from build123d import *

# Parameters (mm, degrees)
SKETCH_1_R      = 17.5
EXTRUDE_1_DEPTH = 10
SKETCH_2_R      = 15
EXTRUDE_2_DEPTH = 300
SKETCH_3_R      = 75
EXTRUDE_3_DEPTH = 10
FILLET_1_R      = 10
HOLE_WIZARD_1_D = 24


with BuildPart() as part:
    # 草图1 → 凸台-拉伸1 (new body)
    with BuildSketch(Plane(origin=(0, 0, 0), x_dir=(1, 0, 0), z_dir=(0, 1, 0))):
        with Locations(Location((0, 0, 0), (0, 0, 270))):
            Circle(SKETCH_1_R)
    extrude(amount=EXTRUDE_1_DEPTH)

    # 草图2 → 凸台-拉伸2 (add)
    with BuildSketch(Plane(origin=(0, 0, 0), x_dir=(1, 0, 0), z_dir=(0, 1, 0))):
        with Locations(Location((0, 0, 0), (0, 0, 270))):
            Circle(SKETCH_2_R)
    extrude(amount=EXTRUDE_2_DEPTH)

    # 草图3 → 凸台-拉伸3 (add)
    with BuildSketch(Plane(origin=(0, 300, 0), x_dir=(1, 0, 0), z_dir=(0, 1, 0))):
        with Locations(Location((0, 0, 0), (0, 0, 270))):
            Circle(SKETCH_3_R)
    extrude(amount=EXTRUDE_3_DEPTH)

    # 圆角1
    fillet_1_edges = [part.edges().sort_by_distance(p)[0] for p in [
        (0, 300, -15),
    ]]
    fillet(fillet_1_edges, radius=FILLET_1_R)

    # 孔1 (through all)
    with Locations(Plane(origin=(0, 310, 0), x_dir=(1, 0, 0), z_dir=(0, 1, 0))):
        with Locations((0, 50), (50, 0), (0, -50), (-50, 0)):
            Hole(HOLE_WIZARD_1_D / 2)


solid = part.part
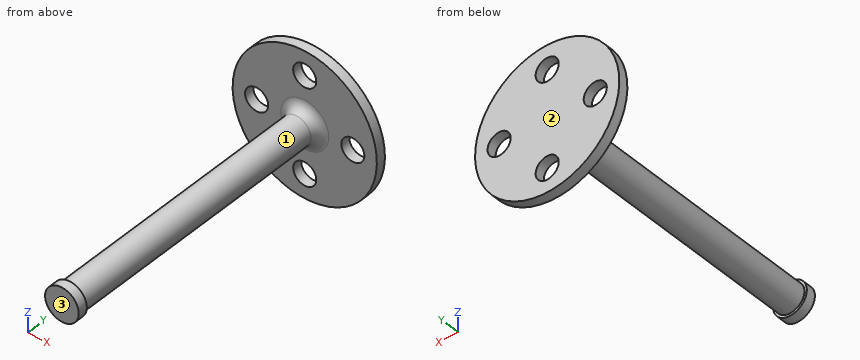
Geometry: final body of the model. Coordinates: model frame, mm. Face numbers are marked on the shaded views. Round coordinates to 2 decimals unless told otherwise and drop trailing zeros. Loops run counter-clockwise (first coordinate to the right, second up) from the corner with the lowest first, then second, coordinate; pieces in that order, holes last. Notation, with made-up numbers: (3.5, -25) - (20.5, -25) arc R12 ccw to (20.5, -14) - close; hole circle Ø7 at (-21.75, -13). An arc over 180 degrees is marked (long way). Write each question's results on one line, items separated by ' | '. Start each with the question number.
1) Mould query, pull axis Y, two halves, no side actions, for the marked faces 1, 2 and 3. Classes: released by +Y, released by -Y, zero draft, split by the parting line, or undercut.
2) Line query: probe 1 along Y at (x, z) = (-25.5, 27.5); probe 2 along X at (y, z) = (164, 1); probe 3 along Z at (x, y) = (-50, 305.5). Output: solid intervals per line, ascending. Write a range as [from, to].
3) Cut plane C-C on x = -50. Return loops of the section in (y, z), then the cut area to 3 significant figures.
4) Cut plane A-A on z = 0. Return loops of the section in (x, y), then the cut area to 3 significant figures.
5) First-contact query: P1, Ø1.5, axis at y = 92, z = -7, coming from the -X side; P2, Ø1.5, axis at x = -4.5, z = 9.5, coming from the -Y side. Flat tips, straight axial feed; report the tip coordinate or a pass-through.
6) Cut plane D-D on z = 50. Return loops of the section in (x, y), then the cut area to 3 significant figures.
7) Cut plane B-B on x = 0. Return loops of the section in (y, z), then the cut area to 3 significant figures.
Verdict:
1) face 1: undercut | face 2: released by +Y | face 3: released by -Y
2) probe 1: y = [300, 310] | probe 2: x = [-14.97, 14.97] | probe 3: z = [-55.9, -12], [12, 55.9]
3) outline: (300, -55.9) - (310, -55.9) - (310, -12) - (300, -12) - close; (300, 12) - (310, 12) - (310, 55.9) - (300, 55.9) - close | area: 878 mm2
4) outline: (-75, 300) - (-62, 300) - (-62, 310) - (-75, 310) - close; (-38, 300) - (-25, 300) arc R10 cw to (-15, 290) - (-15, 10) - (-17.5, 10) - (-17.5, 0) - (17.5, 0) - (17.5, 10) - (15, 10) - (15, 290) arc R10 cw to (25, 300) - (38, 300) - (38, 310) - (-38, 310) - close; (62, 300) - (75, 300) - (75, 310) - (62, 310) - close | area: 10,100 mm2
5) P1: stops at x = -13.64 | P2: stops at y = 0
6) outline: (-55.9, 300) - (-12, 300) - (-12, 310) - (-55.9, 310) - close; (12, 300) - (55.9, 300) - (55.9, 310) - (12, 310) - close | area: 878 mm2
7) outline: (0, -17.5) - (10, -17.5) - (10, -15) - (290, -15) arc R10 cw to (300, -25) - (300, -38) - (310, -38) - (310, 38) - (300, 38) - (300, 25) arc R10 cw to (290, 15) - (10, 15) - (10, 17.5) - (0, 17.5) - close; (300, -75) - (310, -75) - (310, -62) - (300, -62) - close; (300, 62) - (310, 62) - (310, 75) - (300, 75) - close | area: 10,100 mm2
